```python
from build123d import *

# Parameters (mm, degrees)
SALIENTE_EXTRUIR1_DEPTH      = 9
SALIENTE_EXTRUIR1_DEPTH_BACK = 19.5
CROQUIS1_R                   = 12.5
CROQUIS2_R                   = 7
CHAFL_N1_SIZE                = 8
CHAFL_N1_SIZE2               = 12
REDONDEO1_R                  = 1
REDONDEO2_R                  = 1
SALIENTE_EXTRUIR2_START      = -3
SALIENTE_EXTRUIR2_DEPTH      = 12


with BuildPart() as part:
    # Croquis1 → Saliente-Extruir1 (new, two sides: drawn at the far end of the back side and taken through both)
    with BuildSketch(Plane.YZ.offset(-SALIENTE_EXTRUIR1_DEPTH_BACK)):
        with Locations(Location((0, 0, 0), (0, 0, 270))):
            Circle(CROQUIS1_R)
        with BuildLine():
            Line((-1.897366596, 1.3), (1.897366596, 1.3))
            ThreePointArc((1.897366596, 1.3), (0, -2.3), (-1.897366596, 1.3))
        make_face(mode=Mode.SUBTRACT)
    extrude(amount=SALIENTE_EXTRUIR1_DEPTH + SALIENTE_EXTRUIR1_DEPTH_BACK)

    # Croquis2 → Cortar-Revolución1 (revolve, cut)
    with BuildSketch(Plane(origin=(0, 0, 0), x_dir=(-1, 0, 0), z_dir=(0, 1, 0)), mode=Mode.PRIVATE) as cortar_revoluci_n1_sk:
        with Locations((0, 16.2)):
            Circle(CROQUIS2_R)
    revolve(cortar_revoluci_n1_sk.sketch.rotate(Axis((7.517678172, 0, 0), (-1, 0, 0)), 180), axis=Axis((7.517678172, 0, 0), (-1, 0, 0)), mode=Mode.SUBTRACT)

    # Chaflán1
    chafl_n1_edges = [part.edges().sort_by_distance(p)[0] for p in [
        (-19.5, 0, 12.5),
    ]]
    chafl_n1_side = [part.faces().sort_by_distance(p)[0] for p in [
        (-19.5, 0, 12.146446609),
    ]]
    chamfer(chafl_n1_edges, length=CHAFL_N1_SIZE, length2=CHAFL_N1_SIZE2, reference=chafl_n1_side[0])

    # Redondeo1
    redondeo1_edges = [part.edges().sort_by_distance(p)[0] for p in [
        (-7.5, 0, 12.5),
        (-19.5, 0, 4.5),
    ]]
    fillet(redondeo1_edges, radius=REDONDEO1_R)

    # Redondeo2
    redondeo2_edges = [part.edges().sort_by_distance(p)[0] for p in [
        (9, 0, 12.5),
    ]]
    fillet(redondeo2_edges, radius=REDONDEO2_R)

    # Croquis1<3> → Saliente-Extruir2 (add)
    with BuildSketch(Plane.YZ.offset(SALIENTE_EXTRUIR2_START)):
        with BuildLine():
            ThreePointArc((2.3, 0), (2.197037001, 0.680461913), (1.897366596, 1.3))
            Line((1.897366596, 1.3), (-1.897366596, 1.3))
            ThreePointArc((-1.897366596, 1.3), (-0.680461913, -2.197037001), (2.3, 0))
        make_face()
        with BuildLine():
            Line((-1.897366596, 1.3), (1.897366596, 1.3))
            ThreePointArc((1.897366596, 1.3), (0, 2.3), (-1.897366596, 1.3))
        make_face()
    extrude(amount=SALIENTE_EXTRUIR2_DEPTH)


solid = part.part
```
For this review, take the finished solid that the model builds, in its own axes (mm). A direction names the side the tool comes from. Round coordinates to 2 decimals unless told otherwise and drop trailing zeros. Order: outer loops, then holes, each group sorted by start corner. A loop starts at its lowest first (then second) coordinate and runs counter-clockwise, first axis right, second up.
Q1. We need section A-A, the plane x = -4. Give the boundary of the cut face in (y, z).
Findings below:
outline: circle Ø20.91 at (0, 0); hole (-1.9, 1.3) arc R2.3 ccw (long way) to (1.9, 1.3) - close
Q2. Mouldability with a two-part tool opening along Z and no side actions: class faces 3 (the cylindrical face through (6.957, 3.755, -11.923)), 4 (the flat face through (-19.5, 0, 2)), 5 (the flat face through (-11, 0, 1.3)) as pulls with the +Z half, pulls with the -Z half, needs draft (parallel to the pull), parting line crosses it, or undercut.
Findings below:
face 3: parting line crosses it
face 4: needs draft
face 5: undercut
Q3. Wall thickness on line 1 (Y direction, x = -6.75, z = 0); line 2 (Y direction, x = -13.75, z = 0); line 3 (X direction, y = 3.75, z = -9.75): over which ranges is each line inside the solid? List them lowest first.
Findings below:
line 1: y = -12.5 to -2.3, 2.3 to 12.5
line 2: y = -8.33 to -2.3, 2.3 to 8.33
line 3: x = -10.58 to -3.99, 3.99 to 9
Q4. We need section B-B, the plane x = 0. Give the boundary of the cut face in (y, z).
Findings below:
outline: circle Ø18.4 at (0, 0)
Q5. Insertion check: P1, Ø5.5, axis at y = 0, z = 0, coming from the -X side; P2, Ø5, axis at x = -4, z = 5.5, coming from the -Y side; P3, Ø1, axis at x = -3.5, y = -1, coming from the +Z side; P4, Ø1.8, axis at y = 0, z = -0.5, coming from the -X side. Each pin has a flat end and moves straight along its axis. Give the tip position at first contact, or say it passes through.
Findings below:
P1: stops at x = -19.5
P2: stops at y = -11.87
P3: stops at z = 10.41
P4: stops at x = -3
Q6. Machinability: for faces 1 (the cylindrical face through (-6.579, 3.755, -11.923)), 2 (the cylindrical face through (-11.37, 0.07, -2.3)), which of the approach directions +Z, -Z, +X, -X, +Y, -Y give a long, thin tool a straight path to every point of the face, cutting with its end or side? Answer none if there is none.
Findings below:
face 1: +X, -X
face 2: -X
Q7. We need section C-C, the plane x = -10. Give the boundary of the cut face in (y, z), plus the area to 3 significant figures.
Findings below:
outline: circle Ø21.67 at (0, 0); hole (-1.9, 1.3) arc R2.3 ccw (long way) to (1.9, 1.3) - close
area: 355 mm2
